Read the model definition and answer for the solid it produces. Units are mm, in the model's axes. Face numbers are marked on the shaded views. A direction names the side the tool comes from. Round coordinates to 2 decimals unless told otherwise and drop trailing zeros. Write each loop counter-clockwise with the first axis right and the second up, starting at its lowest first coordinate (ties: lowest second). Pieces come first, ordered by that corner, then holes.
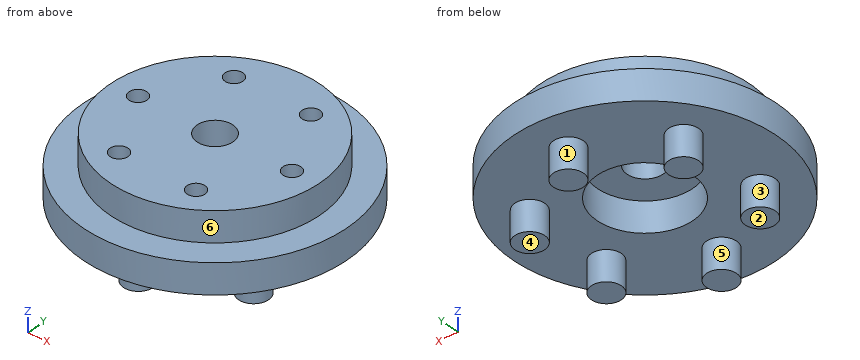
from build123d import *

# Parameters (mm, degrees)
SKETCH1_R           = 22
BOSS_EXTRUDE1_DEPTH = 5
SKETCH2_R           = 17.5
BOSS_EXTRUDE2_DEPTH = 5
SKETCH4_R           = 8
CUT_EXTRUDE2_DEPTH  = 10
SKETCH5_R           = 1.5
CUT_EXTRUDE3_DEPTH  = 3
SKETCH7_R           = 2.5
BOSS_EXTRUDE4_DEPTH = 5
SKETCH8_R           = 8
SKETCH8_R_2         = 3
BOSS_EXTRUDE5_DEPTH = 5


with BuildPart() as part:
    # Sketch1 → Boss-Extrude1 (new body)
    with BuildSketch(Plane.XY):
        Circle(SKETCH1_R)
    extrude(amount=BOSS_EXTRUDE1_DEPTH)

    # Sketch2 → Boss-Extrude2 (add)
    with BuildSketch(Plane.XY.offset(5)):
        Circle(SKETCH2_R)
    extrude(amount=BOSS_EXTRUDE2_DEPTH)

    # Sketch4 → Cut-Extrude2 (cut)
    with BuildSketch(Plane.XY.offset(10)):
        Circle(SKETCH4_R)
    extrude(amount=-CUT_EXTRUDE2_DEPTH, mode=Mode.SUBTRACT)

    # Sketch5 → Cut-Extrude3 (cut)
    with BuildSketch(Plane.XY.offset(10)):
        with Locations((13, 0)):
            Circle(SKETCH5_R)
        with Locations((6.5, -11.258330249)):
            Circle(SKETCH5_R)
        with Locations((-6.5, -11.258330249)):
            Circle(SKETCH5_R)
        with Locations((-13, 0)):
            Circle(SKETCH5_R)
        with Locations((-6.5, 11.258330249)):
            Circle(SKETCH5_R)
        with Locations((6.5, 11.258330249)):
            Circle(SKETCH5_R)
    extrude(amount=-CUT_EXTRUDE3_DEPTH, mode=Mode.SUBTRACT)

    # Sketch7 → Boss-Extrude4 (add)
    with BuildSketch(Plane(origin=(0, 0, 0), x_dir=(-1, 0, 0), z_dir=(0, 0, -1))):
        with Locations(Location((0, 15, 0), (0, 0, 180))):
            Circle(SKETCH7_R)
        with Locations(Location((12.990381057, 7.5, 0), (0, 0, 180))):
            Circle(SKETCH7_R)
        with Locations(Location((12.990381057, -7.5, 0), (0, 0, 180))):
            Circle(SKETCH7_R)
        with Locations(Location((0, -15, 0), (0, 0, 180))):
            Circle(SKETCH7_R)
        with Locations(Location((-12.990381057, -7.5, 0), (0, 0, 180))):
            Circle(SKETCH7_R)
        with Locations(Location((-12.990381057, 7.5, 0), (0, 0, 180))):
            Circle(SKETCH7_R)
    extrude(amount=BOSS_EXTRUDE4_DEPTH)

    # Sketch8 → Boss-Extrude5 (add)
    with BuildSketch(Plane.XY.offset(10)):
        Circle(SKETCH8_R)
        Circle(SKETCH8_R_2, mode=Mode.SUBTRACT)
    extrude(amount=-BOSS_EXTRUDE5_DEPTH)


solid = part.part
Q1. Which of the six approach directions +Z, -Z, +X, -X, +Y, -Y give full straight-line access (tool end or side, diameter ignored) to the marked faces 4, 5 and 6?
Verdict:
face 4: -Z, +X, -X, +Y, -Y
face 5: -Z
face 6: +Z
Q2. Section B-B (z = -2.75) is taken. Determine the outline of the cut face in (x, y), then the cut area to 3 significant figures.
Verdict:
outline: circle Ø5 at (-12.99, -7.5); circle Ø5 at (-12.99, 7.5); circle Ø5 at (0, -15); circle Ø5 at (0, 15); circle Ø5 at (12.99, -7.5); circle Ø5 at (12.99, 7.5)
area: 118 mm2
Q3. Straight lines are drawn through the part: probe 1 along Y at (x, z) = (-6.5, 8.35); probe 2 along Y at (x, z) = (0, 1.45); probe 3 along Z at (x, y) = (7, 5). For each, find the intervals that lie inside material, in ascending order.
Verdict:
probe 1: y = -16.25 to -12.76, -9.76 to 9.76, 12.76 to 16.25
probe 2: y = -22 to -8, 8 to 22
probe 3: z = 0 to 10
Q4. Determine the mould class of the marked faces 1, 2 and 3 for opening direction X: pulls with the +X half, pulls with the -X half, needs draft (parallel to the pull), parting line crosses it, or undercut.
Verdict:
face 1: parting line crosses it
face 2: needs draft
face 3: undercut
Q5. Section A-A (x = 0) is taken. Determine the outline of the cut face in (y, z).
Verdict:
outline: (-22, 0) - (-17.5, 0) - (-17.5, -5) - (-12.5, -5) - (-12.5, 0) - (-8, 0) - (-8, 5) - (-3, 5) - (-3, 10) - (-17.5, 10) - (-17.5, 5) - (-22, 5) - close; (3, 5) - (8, 5) - (8, 0) - (12.5, 0) - (12.5, -5) - (17.5, -5) - (17.5, 0) - (22, 0) - (22, 5) - (17.5, 5) - (17.5, 10) - (3, 10) - close
Q6. Section D-D (x = -6) is taken. Determine the outline of the cut face in (y, z).
Verdict:
outline: (-21.17, 0) - (-5.29, 0) - (-5.29, 5) - (5.29, 5) - (5.29, 0) - (21.17, 0) - (21.17, 5) - (16.44, 5) - (16.44, 10) - (12.67, 10) - (12.67, 7) - (9.84, 7) - (9.84, 10) - (-9.84, 10) - (-9.84, 7) - (-12.67, 7) - (-12.67, 10) - (-16.44, 10) - (-16.44, 5) - (-21.17, 5) - close
Q7. Flat-ended cylindrical pins translate along their axes: pin 1 Ø3.5 at (x, y) = (-6.5, 11.26) entering from -Z; pin 2 Ø0.9 at (x, y) = (6.5, -11.5) entering from +Z; pin 3 Ø4 at (y, z) = (12.5, 3.5) entering from -X. Find the tip coordinate at first contact, or state that the pin passes through.
Verdict:
pin 1: stops at z = 0
pin 2: stops at z = 7
pin 3: stops at x = -19.33
Q8. Section C-C (y = 13.5) is taken. Determine the outline of the cut face in (x, z).
Verdict:
outline: (-17.37, 0) - (-2, 0) - (-2, -5) - (2, -5) - (2, 0) - (17.37, 0) - (17.37, 5) - (11.14, 5) - (11.14, 10) - (-11.14, 10) - (-11.14, 5) - (-17.37, 5) - close
